Geometry check sheet. Reference: the model listing, model coordinates, mm. A direction names the side the tool comes from. Coordinates: 2 decimals unless noted, no trailing zeros. Loops run counter-clockwise (first coordinate to the right, second up) from the corner with the lowest first, then second, coordinate; pieces in that order, holes last. Notation, with made-up numbers: (2, 23.25) - (19, 23.25) arc R20 ccw to (19, 30.25) - close; hole circle Ø3 at (-31.75, 45.5). An arc over 180 degrees is marked (long way). Write item = value, one per line. Start each with the question number.
from build123d import *

# Parameters (mm, degrees)
SKETCH1_R           = 1.778
SKETCH1_R_2         = 3.175
BOSS_EXTRUDE1_DEPTH = 5.461


with BuildPart() as part:
    # Sketch1 → Boss-Extrude1 (new body)
    with BuildSketch(Plane(origin=(0, 0, 0), x_dir=(1, 0, 0), z_dir=(0, 1, 0))):
        with BuildLine():
            Line((-36.075553112, 16.34222836), (-13.499793526, -0.074664302))
            ThreePointArc((-13.499793526, -0.074664302), (7.44200849, -11.263503435), (5.363638877, 12.388760148))
            Line((5.363638877, 12.388760148), (-34.259632886, 29.543416329))
            ThreePointArc((-34.259632886, 29.543416329), (-39.855484626, 29.811728531), (-44.234733225, 26.317772344))
            ThreePointArc((-44.234733225, 26.317772344), (-47.370124011, 20.134748964), (-49.646194202, 13.586469955))
            ThreePointArc((-49.646194202, 13.586469955), (-49.677098428, 12.125807852), (-49.01441114, 10.823757773))
            Line((-49.01441114, 10.823757773), (-48.298660873, 10.002329828))
            ThreePointArc((-48.298660873, 10.002329828), (-46.071262537, 8.895051227), (-43.713289862, 9.687095487))
            Line((-43.713289862, 9.687095487), (-36.075553112, 16.34222836))
        make_face()
        with Locations((-20.862458922, 15.093717491)):
            Circle(SKETCH1_R, mode=Mode.SUBTRACT)
        Circle(SKETCH1_R_2, mode=Mode.SUBTRACT)
        with Locations((-37.413253893, 22.259284205)):
            Circle(SKETCH1_R, mode=Mode.SUBTRACT)
    extrude(amount=BOSS_EXTRUDE1_DEPTH)


solid = part.part
(1) Depth check by flat-ended pin: pin 1 (4 mm diameter, centred on x = -37.41, z = -22.26, fed in from -Y); pin 2 (1.5 mm diameter, centred on x = -16, y = 2.5, fed in from -Z); pin 3 (3 mm diameter, centred on y = 0.5, z = -23, fed in from -X); pin 4 (1.5 mm diameter, centred on y = 1.5, z = -10, fed in from +X). Enter the tip coordinate at first touch or a pass-through.
(2) Scan lines: line 1 (X direction, y = 1.1, z = -16); line 2 (X direction, y = 2.15, z = 0) (3 decimals); line 3 (X direction, y = 5.2, z = 2.5). Record each from-to range of solid material in increasing order.
(3) Sectioned sample at B-B on y = 0.9. Count the separate pieces of the cut face and the enclosed holes in it, plus the area to 3 significant figures.
(4) Sectioned sample at C-C on x = -23.5. Enter the section's corners in (y, z), plus the area to 3 significant figures.
(5) Sectioned sample at D-D on x = -30.5. Enter the section's corners in (y, z), plus the area to 3 significant figures.
(6) Sectioned sample at A-A on x = 0. Enter the section's corners in (y, z) (3 decimals).
(7) Draft check along Z on faces 1 (the face through (-39.948, 2.692, -12.968)), 2 (the face through (-0.69, 2.69, 3.1)), 3 (the face through (-47.332, 2.692, -20.224)). Enter one of: pulls with the +Z half, pulls with the -Z half, needs draft (parallel to the pull), parting line crosses it, or undercut.
(8) Tool access check on faces 4 (the face through (-38.824, 2.692, -21.177)), 5 (the face through (-24.95, 2.69, -8.25)). Record the directions out of +Z, -Z, +X, -X, +Y, -Y that give a thin tool (end or side, any length) a straight path to the whole face; none if there is none.
Working result:
q1.pin_1 = 0
q1.pin_2 = -21.96
q1.pin_3 = -46.77
q1.pin_4 = 9.83
q2.line_1 = -48.92 to -36.47, -35.6 to -22.39, -19.33 to -2.98
q2.line_2 = -13.602 to -3.175, 3.175 to 13.5
q2.line_3 = -13.27 to -1.96, 1.96 to 13.27
q3.separate_pieces = 1
q3.enclosed_holes = 3
q3.area = 1,200 mm2
q4.outline = (0, -24.89) - (5.46, -24.89) - (5.46, -7.2) - (0, -7.2) - close
q4.area = 96.6 mm2
q5.outline = (0, -27.92) - (5.46, -27.92) - (5.46, -12.29) - (0, -12.29) - close
q5.area = 85.3 mm2
q6.outline = (0, -14.711) - (5.461, -14.711) - (5.461, -3.175) - (0, -3.175) - close; (0, 3.175) - (5.461, 3.175) - (5.461, 13.5) - (0, 13.5) - close
q7.face_1 = pulls with the +Z half
q7.face_2 = undercut
q7.face_3 = pulls with the -Z half
q8.face_4 = +Y, -Y
q8.face_5 = +Z, +Y, -Y
